The listing builds one solid part. Answer for the finished solid, in the listing's coordinates (mm). A direction names the side the tool comes from. Give positions to 0.01 mm unless a question says otherwise; leave off trailing zeros. Loops run counter-clockwise (first coordinate to the right, second up) from the corner with the lowest first, then second, coordinate; pieces in that order, holes last. Notation, with made-up numbers: (57.25, 82.25) - (102.25, 82.25) arc R21 ccw to (102.25, 100.25) - close; hole circle Ø10 at (33, -9.5). An arc over 180 degrees is marked (long way). Answer in a Markdown table with one row per item. Add a question column.
```python
from build123d import *

# Parameters (mm, degrees)
BOX001_W                 = 2
BOX001_H                 = 2
BOX001_DEPTH             = 10
CYLINDER_R               = 4
CYLINDER_DEPTH           = 10
CYLINDER_ROLL_ANGLE      = 0.497253
CYLINDER_PITCH_ANGLE     = 0.973542
CYLINDER_PLACEMENT_ANGLE = 0.982028
BOX_W                    = 10
BOX_H                    = 10
BOX_DEPTH                = 10


with BuildPart() as cube001:
    # Box001 → Box001 (new body)
    with BuildSketch(Plane(origin=(23.730946, -3.203472, 0), x_dir=(1, 0, 0), z_dir=(0, 0, 1))):
        with Locations((1, 1)):
            Rectangle(BOX001_W, BOX001_H)
    extrude(amount=BOX001_DEPTH)


with BuildPart() as cylinder:
    # Cylinder → Cylinder (new body)
    with BuildSketch(Plane.XY):
        Circle(CYLINDER_R)
    extrude(amount=CYLINDER_DEPTH)


with BuildPart() as cylinder_1:
    # Cylinder roll: moved
    add(cylinder.part.rotate(Axis((0, 0, 0), (1, 0, 0)), CYLINDER_ROLL_ANGLE))


with BuildPart() as cylinder_2:
    # Cylinder pitch: moved
    add(cylinder_1.part.rotate(Axis((0, 0, 0), (0, 1, 0)), CYLINDER_PITCH_ANGLE))


with BuildPart() as cylinder_3:
    # Cylinder placement: moved
    add(cylinder_2.part.moved(Location((1, 1, 1))).rotate(Axis((1, 1, 1), (0, 0, 1)), CYLINDER_PLACEMENT_ANGLE))


with BuildPart() as cut001:
    # Box → Box (new body)
    with BuildSketch(Plane(origin=(-0.44599, 0.596456, 0), x_dir=(1, 0, 0), z_dir=(0, 0, 1))):
        with Locations((5, 5)):
            Rectangle(BOX_W, BOX_H)
    extrude(amount=BOX_DEPTH)

    # Cut: cut Cylinder
    add(cylinder_3.part, mode=Mode.SUBTRACT)


with BuildPart() as cut001_1:
    # Cut placement: moved
    add(cut001.part.moved(Location((17.420948, -9.267728, 0))))

    # Cut001: cut Cube001
    add(cube001.part, mode=Mode.SUBTRACT)


solid = cut001_1.part
```
(1) The mould has two halves that part along X. Classify faces 1 (the face through (25, -1.203, 5)), 2 (the face through (26.975, -4, 5)), 3 (the face through (22, -4, 0)): pulls with the +X half, pulls with the -X half, needs draft (parallel to the pull), parting line crosses it, or undercut.
(2) A cutting plane is placed at B-B on y = -2.5. Determine the outline of the cut face in (x, z).
(3) Find the intervals of material crossed by line 1 along X through (y, z) = (-2.75, 2); line 2 along Y through (x, z) = (25, 3); line 3 along Y through (x, z) = (18.5, 5.5), in increasing order. Write a range as [from, to].
(4) A tool of negligible diameter and unlimited length cuts with its end or side. For faces 4 (the face through (25.731, -2, 5)), 5 (the face through (22, 1.329, 5)), from which of +Z, -Z, +X, -X, +Y, -Y can it reach the whole face along a straight path? Write none if from no direction.
(5) A cutting plane is placed at A-A on x = 25.5. Determine the outline of the cut face in (y, z), plus the area to 3 significant figures.
Evaluation:
| question | item | result |
|---|---|---|
| 1 | face 1 | undercut |
| 1 | face 2 | pulls with the +X half |
| 1 | face 3 | needs draft |
| 2 | outline | (16.97, 0) - (23.73, 0) - (23.73, 10) - (16.97, 10) - close; (25.73, 0) - (26.97, 0) - (26.97, 10) - (25.73, 10) - close |
| 3 | line 1 | x = [16.97, 23.73], [25.73, 26.97] |
| 3 | line 2 | y = [-8.67, -3.2], [-1.2, 1.33] |
| 3 | line 3 | y = [-4.31, 1.33] |
| 4 | face 4 | +Z, -Z |
| 4 | face 5 | +Z, -Z, +X, -X, +Y |
| 5 | outline | (-8.67, 0) - (-3.2, 0) - (-3.2, 10) - (-8.67, 10) - close; (-1.2, 0) - (1.33, 0) - (1.33, 10) - (-1.2, 10) - close |
| 5 | area | 80.0 mm² |
